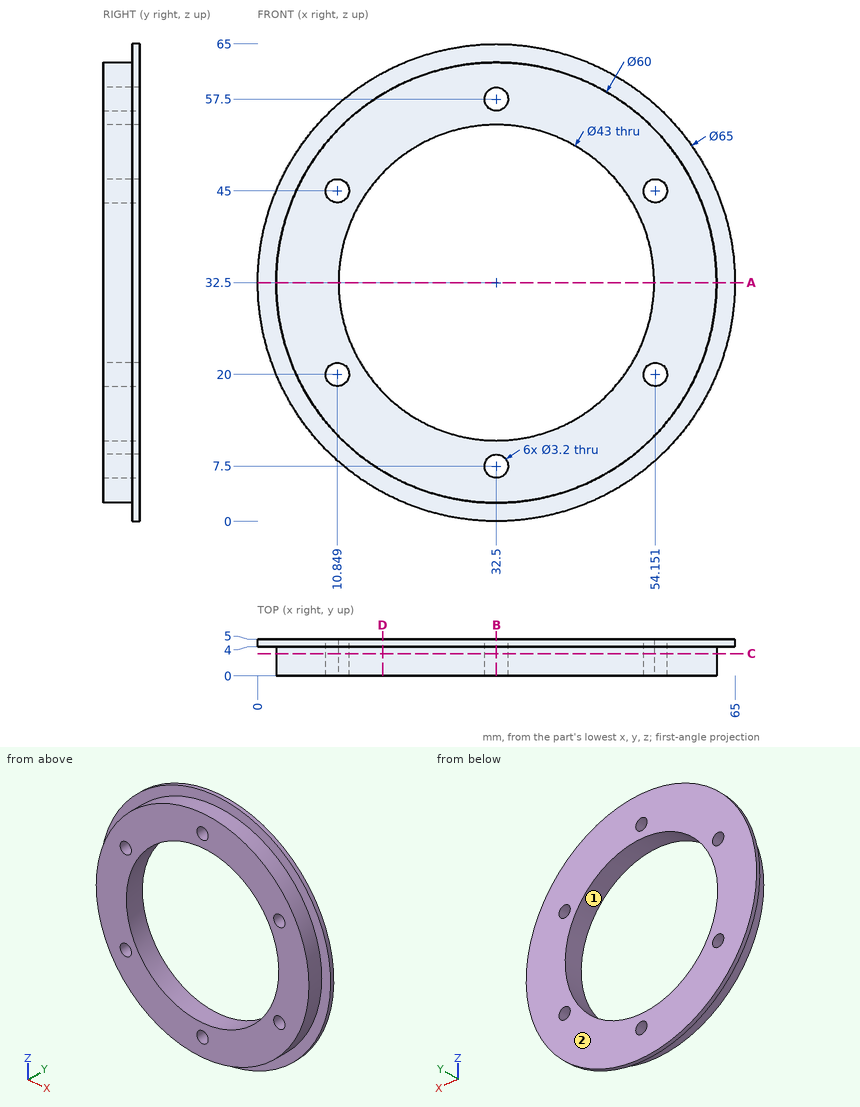
The drawing under review shows one solid part. Ordinate dimensions are in mm from its lowest x, y, z. Give positions to 0.01 mm unless a question says otherwise; leave off trailing zeros. Loops run counter-clockwise (first coordinate to the right, second up) from the corner with the lowest first, then second, coordinate; pieces in that order, holes last. Notation, with made-up numbers: M 10.25,64 L 40.25,64 A22 ccw 40.25,101 Z; hole C 0.25,-5.5 d10. An arc over 180 degrees is marked long. Return JSON: item names as keys, results as strings. Group by question number.
Item 1: We need section C-C (y = 3.05). Give the boundary of the cut face in (x, z).
Item 2: For probe 1 along X at (y, z) = (3.2, 45); probe 2 along Y at (x, z) = (46, 61); probe 3 along X at (y, z) = (3.9, 46) (1 decimal), list the stretches that pass through material, from the lowest coordinate up.
Item 3: Insertion check: pin 1 Ø2 at (y, z) = (3.5, 29.5) entering from +X; pin 2 Ø1.5 at (x, y) = (52, 4) entering from +Z (1 decimal); pin 3 Ø3 at (x, y) = (52.5, 2) entering from +Z. Each pin has a flat end and moves straight along its axis. Give the tip position at first contact, or say it passes through.
Item 4: Mouldability with a two-part tool opening along X and no side actions: class the marked faces 1 and 2 as released by +X, released by -X, zero draft, split by the parting line, or undercut.
Item 5: We need section A-A (z = 32.5). Give the boundary of the cut face in (x, y), and give its area (3 significant figures).
Item 6: We need section D-D (x = 17). Give the boundary of the cut face in (y, z) (1 decimal).
Item 7: We need section B-B (x = 32.5). Give the boundary of the cut face in (y, z).
Output:
{
 "1": {"outline": "C 32.5,32.5 d60; hole C 10.85,20 d3.2; hole C 10.85,45 d3.2; hole C 32.5,32.5 d43; hole C 32.5,7.5 d3.2; hole C 32.5,57.5 d3.2; hole C 54.15,20 d3.2; hole C 54.15,45 d3.2"},
 "2": {"probe 1": "x = 5.23 to 9.25, 12.45 to 15.01, 49.99 to 52.55, 55.75 to 59.77", "probe 2": "y = 4 to 5", "probe 3": "x = 5.7 to 9.6, 12.1 to 15.8, 49.2 to 52.9, 55.4 to 59.3"},
 "3": {"pin 1": "stops at x = 64.93", "pin 2": "stops at z = 59", "pin 3": "stops at z = 56.12"},
 "4": {"face 1": "undercut", "face 2": "zero draft"},
 "5": {"outline": "M 0,4 L 2.5,4 L 2.5,0 L 11,0 L 11,5 L 0,5 Z; M 54,0 L 62.5,0 L 62.5,4 L 65,4 L 65,5 L 54,5 Z", "area": "90.0 mm^2"},
 "6": {"outline": "M 0,6.8 L 4,6.8 L 4,3.9 L 5,3.9 L 5,17.6 L 0,17.6 Z; M 0,47.4 L 5,47.4 L 5,61.1 L 4,61.1 L 4,58.2 L 0,58.2 Z"},
 "7": {"outline": "M 0,2.5 L 4,2.5 L 4,0 L 5,0 L 5,5.9 L 0,5.9 Z; M 0,9.1 L 5,9.1 L 5,11 L 0,11 Z; M 0,54 L 5,54 L 5,55.9 L 0,55.9 Z; M 0,59.1 L 5,59.1 L 5,65 L 4,65 L 4,62.5 L 0,62.5 Z"}
}
